```python
from build123d import *

# Parameters (mm, degrees)
ESQUISSE2_W                  = 100
ESQUISSE2_H                  = 100
BOSS_EXTRU_1_DEPTH           = 51
BOSS_EXTRU_1_TAPER           = 20
ENL_V_MAT_EXTRU_1_DEPTH      = 140.622233322
ENL_V_MAT_EXTRU_1_DEPTH_BACK = 140.622233322
ESQUISSE3_R                  = 25
ENL_V_MAT_EXTRU_2_DEPTH      = 140.622233322
ENL_V_MAT_EXTRU_2_DEPTH_BACK = 10
ESQUISSE5_R                  = 35
ENL_V_START                  = -10
ESQUISSE6_R                  = 35
ENL_V_MAT_EXTRU_3_DEPTH      = 10
ESQUISSE7_W                  = 50
ESQUISSE7_H                  = 50
ENL_V_MAT_EXTRU_4_DEPTH      = 140.622233322
CONG_1_R                     = 15
ENL_V_MAT_EXTRU_8_DEPTH      = 10
BOSS_EXTRU_2_DEPTH           = 10


with BuildPart() as part:
    # Esquisse2 → Boss.-Extru.1 (new body)
    with BuildSketch(Plane.XY):
        with Locations((-23.410404624, -10.838150289)):
            Rectangle(ESQUISSE2_W, ESQUISSE2_H)
    boss_extru_1 = extrude(amount=BOSS_EXTRU_1_DEPTH, taper=BOSS_EXTRU_1_TAPER)

    # Symétrie4: Boss.-Extru.1 across plane
    add(boss_extru_1.mirror(Plane.XY.offset(51)))

    # Esquisse3 → Enlèv. mat.-Extru.1 (cut, two sides: drawn at the far end of the back side and taken through both)
    with BuildSketch(Plane.XY.offset(102).offset(-ENL_V_MAT_EXTRU_1_DEPTH_BACK)):
        with Locations((-23.410404624, -10.838150289)):
            Circle(ESQUISSE3_R)
    extrude(amount=ENL_V_MAT_EXTRU_1_DEPTH + ENL_V_MAT_EXTRU_1_DEPTH_BACK, mode=Mode.SUBTRACT)

    # Esquisse5 → Enlèv. mat.-Extru.2 (cut, two sides: drawn at the far end of the back side and taken through both)
    with BuildSketch(Plane.XY.offset(102).offset(-ENL_V_MAT_EXTRU_2_DEPTH_BACK)):
        with Locations(Location((-23.410404624, -10.838150289, 0), (0, 0, 180))):
            Circle(ESQUISSE5_R)
    extrude(amount=ENL_V_MAT_EXTRU_2_DEPTH + ENL_V_MAT_EXTRU_2_DEPTH_BACK, mode=Mode.SUBTRACT)

    # Esquisse6 → Enlèv. mat.-Extru.3 (cut)
    with BuildSketch(Plane(origin=(0, 0, 0), x_dir=(-1, 0, 0), z_dir=(0, 0, -1)).offset(ENL_V_START)):
        with Locations((23.410404624, -10.838150289)):
            Circle(ESQUISSE6_R)
    extrude(amount=ENL_V_MAT_EXTRU_3_DEPTH, mode=Mode.SUBTRACT)

    # Esquisse7 → Enlèv. mat.-Extru.4 (cut, through all)
    with BuildSketch(Plane(origin=(0, 0, 0), x_dir=(-1, 0, 0), z_dir=(0, 0, -1))):
        with Locations((48.410404624, -35.838150289)):
            Rectangle(ESQUISSE7_W, ESQUISSE7_H)
    extrude(amount=-ENL_V_MAT_EXTRU_4_DEPTH, mode=Mode.SUBTRACT)

    # Congé1
    cong_1_edges = [part.edges().sort_by_distance(p)[0] for p in [
        (8.027113428, -10.838150289, 51),
        (-23.410404624, 20.599367763, 51),
        (-54.847922677, 4.880608737, 51),
    ]]
    fillet(cong_1_edges, radius=CONG_1_R)

    # Esquisse8 → Enlèv. mat.-Extru.8 (cut)
    with BuildSketch(Plane(origin=(0, 0, 0), x_dir=(-1, 0, 0), z_dir=(0, 0, -1))):
        with BuildLine():
            Line((-15.12691495, 31.941809973), (-4.520313233, 21.335208255))
            ThreePointArc((-4.520313233, 21.335208255), (-4.520313233, 17.092567568), (-8.76295392, 17.092567568))
            Line((-8.76295392, 17.092567568), (-19.369555638, 27.699169286))
            ThreePointArc((-19.369555638, 27.699169286), (-19.369555638, 31.941809973), (-15.12691495, 31.941809973))
        make_face()
        with BuildLine():
            Line((-19.369555638, -49.375469864), (-8.76295392, -38.768868146))
            ThreePointArc((-8.76295392, -38.768868146), (-4.520313233, -38.768868146), (-4.520313233, -43.011508833))
            Line((-4.520313233, -43.011508833), (-15.12691495, -53.618110551))
            ThreePointArc((-15.12691495, -53.618110551), (-19.369555638, -53.618110551), (-19.369555638, -49.375469864))
        make_face()
        with BuildLine():
            Line((51.341122481, 21.335208255), (61.947724199, 31.941809973))
            ThreePointArc((61.947724199, 31.941809973), (66.190364886, 31.941809973), (66.190364886, 27.699169286))
            Line((66.190364886, 27.699169286), (55.583763168, 17.092567568))
            ThreePointArc((55.583763168, 17.092567568), (51.341122481, 17.092567568), (51.341122481, 21.335208255))
        make_face()
    extrude(amount=-ENL_V_MAT_EXTRU_8_DEPTH, mode=Mode.SUBTRACT)

    # Esquisse9 → Boss.-Extru.2 (add)
    with BuildSketch(Plane(origin=(0, 0, 0), x_dir=(-1, 0, 0), z_dir=(0, 0, -1))):
        Polygon((-26.589595376, -60.838150289), (23.410404624, -60.838150289), (23.410404624, -57.838150289), (-23.589595376, -57.838150289), (-23.589595376, 36.161849711), (70.410404624, 36.161849711), (70.410404624, -10.838150289), (73.410404624, -10.838150289), (73.410404624, 39.161849711), (-26.589595376, 39.161849711), align=None)
    extrude(amount=BOSS_EXTRU_2_DEPTH)


solid = part.part
```
Here's how the part is built. I have some questions about the finished solid (model axes, mm). A direction names the side the tool comes from. Round coordinates to 2 decimals unless told otherwise and drop trailing zeros. Loops run counter-clockwise (first coordinate to the right, second up) from the corner with the lowest first, then second, coordinate; pieces in that order, holes last. Notation, with made-up numbers: (75, 89.5) -> (106, 89.5) arc R6 ccw to (106, 95.5) -> close; hole circle Ø8 at (-6, 71). An arc over 180 degrees is marked (long way). Answer as CSV lines item,"result".
1. Thinking about a two-plate mould opening in Z: for faces 6 (the face through (18.36, -10.14, 22.61)), 7 (the face through (25, 1, -10)), 8 (the face through (0, -57.838, -5)), which applies, released by +Z, released by -Z, zero draft, split by the parting line, or undercut?
Final values:
face 6,"undercut"
face 7,"released by -Z"
face 8,"zero draft"
2. If we section it at B-B on y = -4.5: Please give me the cut outline in (x, z).
Final values:
outline,"(-73.41, -10) -> (-70.41, -10) -> (-70.41, 0) -> (-57.83, 0) -> (-57.83, 10) -> (-47.59, 10) -> (-47.59, 92) -> (-57.83, 92) -> (-57.83, 102) -> (-73.41, 102) -> (-56.72, 56.13) arc R15 cw to (-56.72, 45.87) -> (-73.41, 0) -> close; (0.77, 10) -> (11.01, 10) -> (11.01, 0) -> (23.59, 0) -> (23.59, -10) -> (26.59, -10) -> (26.59, 0) -> (9.89, 45.87) arc R15 cw to (9.89, 56.13) -> (26.59, 102) -> (11.01, 102) -> (11.01, 92) -> (0.77, 92) -> close"
3. For pin 1 (8.5 mm diameter, centred on x = 9.5, y = -49.5, fed in from -Z); pin 2 (6 mm diameter, centred on x = -60.5, z = 78, fed in from +Y); pin 3 (5 mm diameter, centred on x = -49, z = 6, fed in from +Y), each with a flat end and sliding along its axis, tell me the tip position at first contact or that it passes through.
Final values:
pin 1,"stops at z = 0"
pin 2,"stops at y = 31.52"
pin 3,"stops at y = 37.89"
4. If we section it at D-D on z = 1.5: Please give me the cut outline in (x, y).
Final values:
outline,"(-72.86, -10.84) -> (-58.41, -10.84) arc R35 cw (long way) to (-23.41, -45.84) -> (-23.41, -60.29) -> (26.04, -60.29) -> (26.04, 38.62) -> (-72.86, 38.62) -> close; hole (-66.19, 27.7) -> (-55.58, 17.09) arc R3 ccw to (-51.34, 21.34) -> (-61.95, 31.94) arc R3 ccw to start; hole (4.52, -43.01) -> (15.13, -53.62) arc R3 ccw to (19.37, -49.38) -> (8.76, -38.77) arc R3 ccw to start; hole (4.52, 21.34) arc R3 ccw to (8.76, 17.09) -> (19.37, 27.7) arc R3 ccw to (15.13, 31.94) -> close"
5. If we section it at A-A on x = -12: Please give me the cut outline in (y, z), plus the area to 3 significant figures.
Final values:
outline,"(-60.84, -10) -> (-57.84, -10) -> (-57.84, 0) -> (-43.93, 0) -> (-43.93, 10) -> (-33.08, 10) -> (-33.08, 92) -> (-43.93, 92) -> (-43.93, 102) -> (-60.84, 102) -> (-42.28, 51) -> (-60.84, 0) -> close; (11.41, 10) -> (22.25, 10) -> (22.25, 0) -> (36.16, 0) -> (36.16, -10) -> (39.16, -10) -> (39.16, 0) -> (22.47, 45.87) arc R15 cw to (22.47, 56.13) -> (39.16, 102) -> (22.25, 102) -> (22.25, 92) -> (11.41, 92) -> close"
area,"3,400 mm^2"
6. If we section it at C-C on z = 36: Please give me the cut outline in (x, y).
Final values:
outline,"(-60.31, -10.84) -> (-48.41, -10.84) arc R25 cw (long way) to (-23.41, -35.84) -> (-23.41, -47.74) -> (13.49, -47.74) -> (13.49, 26.06) -> (-60.31, 26.06) -> close"
7. If I drill on L1, parallel to X at y = 16, z = -4; L2, parallel to Z at x = -22, y = 15.5; L3, parallel to Y at x = -16.5, z = 46.5, over which ranges is the centre line in solid material (lowest first)?
Final values:
L1,"x = -73.41 to -70.41, 23.59 to 26.59"
L2,"z = 10 to 92"
L3,"y = -43.91 to -34.86, 13.19 to 22.25"
8. Which directions (+Z, -Z, +X, -X, +Y, -Y) give clear straight access to the entire face, cutting with the end or side of a thin tool? Please do faces 1 (the face through (-23.41, -43, 47)), 2 (the face through (-65.18, 8.26, 22.61)), 3 (the face through (2.14, 13.08, 96.93)), 4 (the face through (-60.96, 22.47, 4.93)), 5 (the face through (-3.62, -51.69, 76.86)).
Final values:
face 1,"+Z, -Z, -X, -Y"
face 2,"-X, +Y, -Y"
face 3,"+Z"
face 4,"-Z"
face 5,"+X, -X, -Y"
